Part print with two shaded views. Sizes in mm from the minimum x, y, z corner. A direction names the side the tool comes from. Round coordinates to 2 decimals unless told otherwise and drop trailing zeros. Write each loop counter-clockwise with the first axis right and the second up, starting at its lowest first coordinate (ties: lowest second). Pieces come first, ordered by that corner, then holes. Notation, with made-up numbers: (89, 33) -> (137, 33) arc R26 ccw to (137, 60) -> close; hole circle Ø8 at (65.5, -28.5). An arc over 180 degrees is marked (long way). Answer in a Markdown table with one row per item.
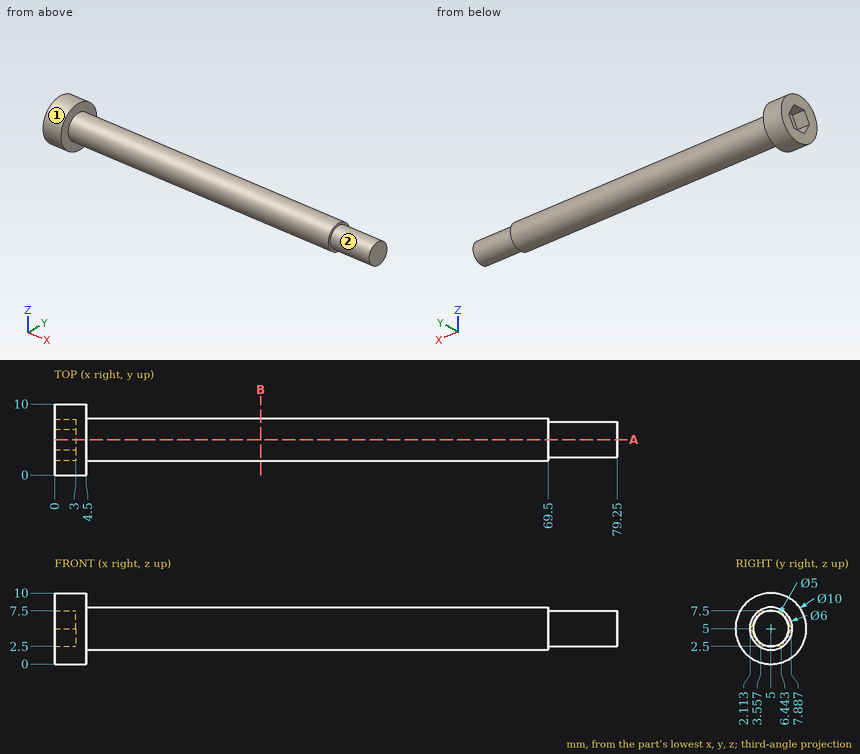
Q1. Wall check: line 1 (X direction, y = 7.25, z = 1.75); line 2 (X direction, y = 2.5, z = 3.5); line 3 (Y direction, x = 70, z = 4.75). Give the ranges that are in metal, low to high. Write a range as [from, to].
A:
| item | result |
|---|---|
| line 1 | [0, 4.5] |
| line 2 | [0, 69.5] |
| line 3 | [2.51, 7.49] |
Q2. Saw through at B-B on x = 29. Write the cut outline in (y, z), plus the area to 3 significant figures.
A:
| item | result |
|---|---|
| outline | circle Ø6 at (5, 5) |
| area | 28.3 mm² |
Q3. Saw through at A-A on y = 5. Write the cut outline in (x, z).
A:
| item | result |
|---|---|
| outline | (0, 0) -> (4.5, 0) -> (4.5, 2) -> (69.5, 2) -> (69.5, 2.5) -> (79.25, 2.5) -> (79.25, 7.5) -> (69.5, 7.5) -> (69.5, 8) -> (4.5, 8) -> (4.5, 10) -> (0, 10) -> (0, 7.5) -> (3, 7.5) -> (3, 2.5) -> (0, 2.5) -> close |
Q4. Drop flat-ended pins along their axis: P1, Ø1.5, axis at x = 23.5, z = 1.5, coming from the +Y side; P2, Ø1.5, axis at y = 5.5, z = 4.5, coming from the -X side; P3, Ø1, axis at x = 33.5, z = 7.5, coming from the -Y side (1 decimal). Give the stop position or say it passes through.
A:
| item | result |
|---|---|
| P1 | y = 6.2 |
| P2 | x = 3 |
| P3 | y = 2.8 |
Q5. Which spindle directions (+Z, -Z, +X, -X, +Y, -Y) get a long thin tool onto all of the face, cutting with end or side? Do the marked faces 1 and 2. Say none if no direction does.
A:
| item | result |
|---|---|
| face 1 | +X, -X |
| face 2 | +X |
